Work out the finished part from the listing and answer in its coordinate system (mm). A direction names the side the tool comes from. Round coordinates to 2 decimals unless told otherwise and drop trailing zeros. Order: outer loops, then holes, each group sorted by start corner. A loop starts at its lowest first (then second) coordinate and runs counter-clockwise, first axis right, second up. Notation, with made-up numbers: (-4, 63) - (52, 63) arc R18 cw to (52, 70) - close; hole circle Ø11 at (-39, 58.5). An arc over 180 degrees is marked (long way). Use CSV: the item, a comma, the result in double quotes.
Autodesk Inventor part; units mm, degrees
ref_plane "YZ Plane" through (0, 0, 0) normal (1, 0, 0) x (0, 1, 0)
ref_plane "XZ Plane" through (0, 0, 0) normal (0, 1, 0) x (-1, 0, 0)
ref_plane "XY Plane" through (0, 0, 0) normal (0, 0, 1) x (1, 0, 0)
sketch "スケッチ1" plane through (0, 0, 0) normal (0, 0, 1) x (1, 0, 0)
  line L0 (0, 0) -> (50, 0)
  line L1 (50, 0) -> (50, 53)
  line L2 (50, 53) -> (0, 53)
  line L3 (0, 53) -> (0, 0)
  line L4 (1.5, 2) -> (48.5, 2)
  line L5 (48.5, 2) -> (48.5, 7)
  line L6 (48.5, 7) -> (1.5, 7)
  line L7 (1.5, 7) -> (1.5, 2)
  line L8 (1.5, 51) -> (48.5, 51)
  line L9 (48.5, 51) -> (48.5, 44)
  line L10 (48.5, 44) -> (1.5, 44)
  line L11 (1.5, 44) -> (1.5, 51)
  line L12 (0, 27) -> (1.5, 27)
  line L13 (1.5, 27) -> (1.5, 22)
  line L14 (1.5, 22) -> (0, 22)
  line L15 (50, 27) -> (48.5, 27)
  line L16 (48.5, 27) -> (48.5, 22)
  line L17 (48.5, 22) -> (50, 22)
  dimension "d0" = 50
  dimension "d1" = 53
  dimension "d2" = 2
  dimension "d3" = 1.5
  dimension "d4" = 1.5
  dimension "d5" = 5
  dimension "d6" = 2
  dimension "d7" = 7
  dimension "d8" = 5
  dimension "d9" = 17
extrude "押し出し1" add sketch "スケッチ1" along normal blind 20.1 contours L3 L14 L13 L12 L2 L1 L15 L16 L17 L0
fillet "フィレット1" radius 5 8 edges at (0.75, 27, 20.1) (0.75, 27, 0) (0.75, 22, 0) (0.75, 22, 20.1) (49.25, 22, 0) (49.25, 22, 20.1) (49.25, 27, 0) (49.25, 27, 20.1)
properties part number "サーボ"
(1) Find section C-C (y = 25). Determine the outline of the cut face in (x, z), and give its area (3 significant figures).
Findings below:
outline,"(1.5, 0) - (48.5, 0) - (48.5, 20.1) - (1.5, 20.1) - close"
area,"945 mm²"
(2) This flat-tipped pin is pushed along its axis until it touches: pin 1 (2 mm diameter, centred on y = 46.5, z = 13.5, fed in from -X). Where does it stop, or does it pass through?
Findings below:
pin 1,"stops at x = 0"
(3) Find the intervals of material crossed by L1, parallel to Y at x = 32, z = 1.75; L2, parallel to X at y = 49, z = 19; L3, parallel to X at y = 26.5, z = 7.75, in increasing order. Write a range as from..to.
Findings below:
L1,"y = 0..2, 7..44, 51..53"
L2,"x = 0..1.5, 48.5..50"
L3,"x = 1.5..48.5"
(4) Find section B-B (x = 9.5). Determine the outline of the cut face in (y, z).
Findings below:
outline,"(0, 0) - (2, 0) - (2, 20.1) - (0, 20.1) - close; (7, 0) - (44, 0) - (44, 20.1) - (7, 20.1) - close; (51, 0) - (53, 0) - (53, 20.1) - (51, 20.1) - close"
(5) Find section A-A (z = 7.5). Determine the outline of the cut face in (x, y).
Findings below:
outline,"(0, 0) - (50, 0) - (50, 22) - (48.5, 22) - (48.5, 27) - (50, 27) - (50, 53) - (0, 53) - (0, 27) - (1.5, 27) - (1.5, 22) - (0, 22) - close; hole (1.5, 2) - (48.5, 2) - (48.5, 7) - (1.5, 7) - close; hole (1.5, 44) - (48.5, 44) - (48.5, 51) - (1.5, 51) - close"
(6) Find section D-D (z = 3.25). Determine the outline of the cut face in (x, y).
Findings below:
outline,"(0, 0) - (50, 0) - (50, 21.68) - (48.5, 21.68) - (48.5, 27.32) - (50, 27.32) - (50, 53) - (0, 53) - (0, 27.32) - (1.5, 27.32) - (1.5, 21.68) - (0, 21.68) - close; hole (1.5, 2) - (48.5, 2) - (48.5, 7) - (1.5, 7) - close; hole (1.5, 44) - (48.5, 44) - (48.5, 51) - (1.5, 51) - close"
(7) The mould has two halves that part along Y. Classify faces 1 (the cylindrical face through (49, 20, 1)), 2 (the flat face through (0, 11, 10)): released by +Y, released by -Y, zero draft, split by the parting line, or undercut.
Findings below:
face 1,"undercut"
face 2,"zero draft"
(8) For faces 3 (the flat face through (48.5, 4, 10)), 4 (the cylindrical face through (49, 29, 1)), 5 (the cylindrical face through (1, 21, 2)), determine the directions among +Z, -Z, +X, -X, +Y, -Y from which every point of the face is accessible in a straight line to the end or side of a thin tool.
Findings below:
face 3,"+Z, -Z"
face 4,"-Z, +X"
face 5,"-Z, -X"
